The model under review builds one solid part; all positions refer to its coordinate system, in mm. A direction names the side the tool comes from. Round coordinates to 2 decimals unless told otherwise and drop trailing zeros. Write each loop counter-clockwise with the first axis right and the second up, starting at its lowest first coordinate (ties: lowest second). Pieces come first, ordered by that corner, then holes. Notation, with made-up numbers: (46, 79) -> (52, 79) arc R18 cw to (52, 85) -> close; hole circle Ø11 at (39, -32). An arc over 180 degrees is marked (long way). Answer as a JSON object with one key per item and string values. Group by question number.
1) We need section D-D, the plane z = 1.6. Write out the cut boundary in (x, y), then the cut area to 3 significant figures.
2) We need section B-B, the plane z = 0.5. Write out the cut boundary in (x, y).
3) Insertion check: pin 1 Ø3 at (x, z) = (5.5, 0.5) entering from -Y; pin 2 Ø1.1 at (x, z) = (7.54, 0) entering from +Y; pin 3 Ø0.6 at (x, z) = (-9, 0) entering from +Y. Each pin has a flat end and moves straight along its axis. Give the tip position at first contact, or say it passes through.
4) Mouldability with a two-part tool opening along X and no side actions: class faces 4 (the flat face through (11, 5, 0)), 5 (the flat face through (11, 0, 1)), 6 (the flat face through (0, 5, 0)) as pulls with the +X half, pulls with the -X half, needs draft (parallel to the pull), parting line crosses it, or undercut.
5) We need section C-C, the plane y = 2.25. Write out the cut boundary in (x, z) (3 decimals).
6) To check wall thickness, follow probe 1 along X at (y, z) = (1.7, 0) (3 decimals); probe 2 along Z at (x, y) = (-11.5, 3) (3 decimals); probe 3 along Y at (x, z) = (3.5, -1.9). State the ranges of each line that lie inside material, in increasing order. Write a range as [from, to].
7) We need section A-A, the plane y = 6.5. Write out the cut boundary in (x, z) (3 decimals), then the cut area to 3 significant figures.
8) Machinability: for faces 1 (the flat face through (-12, 0, 1)), 2 (the cylindrical face through (-7.628, 6.521, -0.263)), 3 (the cylindrical face through (10.626, 2.465, -0.038)), which of the approach directions +Z, -Z, +X, -X, +Y, -Y give a long, thin tool a straight path to every point of the face, cutting with its end or side? Answer none if there is none.
from build123d import *

# Parameters (mm, degrees)
SKETCH1_R             = 2.875
SKETCH1_R_2           = 0.875
BOSS_EXTRUDE1_DEPTH   = 5
BOSS_EXTRUDE1_2_DEPTH = 5
BOSS_EXTRUDE2_DEPTH   = 3
SKETCH3_R             = 0.875
CUT_EXTRUDE1_DEPTH    = 3


with BuildPart() as part:
    # Sketch1 → Boss-Extrude1 (new body)
    with BuildSketch(Plane(origin=(0, 0, 0), x_dir=(1, 0, 0), z_dir=(0, 1, 0))):
        with Locations((-11.5, 0)):
            Circle(SKETCH1_R)
        with Locations((-11.5, 0)):
            Circle(SKETCH1_R_2, mode=Mode.SUBTRACT)
    extrude(amount=BOSS_EXTRUDE1_DEPTH)



with BuildPart() as body_2:
    # Sketch1 → Boss-Extrude1 2 (new body)
    with BuildSketch(Plane(origin=(0, 0, 0), x_dir=(1, 0, 0), z_dir=(0, 1, 0))):
        with Locations((11.5, 0)):
            Circle(SKETCH1_R)
        with Locations((11.5, 0)):
            Circle(SKETCH1_R_2, mode=Mode.SUBTRACT)
    extrude(amount=BOSS_EXTRUDE1_2_DEPTH)


with BuildPart() as part_1:
    add(part.part)

    add(body_2.part)  # Boss-Extrude2 merges body 2
    # Sketch2 → Boss-Extrude2 (add)
    with BuildSketch(Plane(origin=(0, 5, 0), x_dir=(1, 0, 0), z_dir=(0, 1, 0))):
        with BuildLine():
            ThreePointArc((-10.625, 0), (-10.881281566, 0.618718434), (-11.5, 0.875))
            Line((-11.5, 0.875), (-11.5, -0.875))
            ThreePointArc((-11.5, -0.875), (-10.881281566, -0.618718434), (-10.625, 0))
        make_face()
        with BuildLine():
            Line((-11.5, -0.875), (-11.5, 0.875))
            ThreePointArc((-11.5, 0.875), (-12.375, 0), (-11.5, -0.875))
        make_face()
        with BuildLine():
            ThreePointArc((-8.625, 0), (-9.467068004, 2.032931996), (-11.5, 2.875))
            Line((-11.5, 2.875), (-11.5, 0.875))
            ThreePointArc((-11.5, 0.875), (-10.881281566, 0.618718434), (-10.625, 0))
            ThreePointArc((-10.625, 0), (-10.881281566, -0.618718434), (-11.5, -0.875))
            Line((-11.5, -0.875), (-11.5, -2.875))
            ThreePointArc((-11.5, -2.875), (-9.467068004, -2.032931996), (-8.625, 0))
        make_face()
        with BuildLine():
            Line((-11.5, 0.875), (-11.5, 2.875))
            ThreePointArc((-11.5, 2.875), (-14.375, 0), (-11.5, -2.875))
            Line((-11.5, -2.875), (-11.5, -0.875))
            ThreePointArc((-11.5, -0.875), (-12.375, 0), (-11.5, 0.875))
        make_face()
        with BuildLine():
            Line((11.5, 2.875), (-11.5, 2.875))
            ThreePointArc((-11.5, 2.875), (-9.467068004, 2.032931996), (-8.625, 0))
            ThreePointArc((-8.625, 0), (-9.467068004, -2.032931996), (-11.5, -2.875))
            Line((-11.5, -2.875), (11.5, -2.875))
            ThreePointArc((11.5, -2.875), (8.625, 0), (11.5, 2.875))
        make_face()
        with BuildLine():
            ThreePointArc((14.375, 0), (13.532931996, 2.032931996), (11.5, 2.875))
            Line((11.5, 2.875), (11.5, -2.875))
            ThreePointArc((11.5, -2.875), (13.532931996, -2.032931996), (14.375, 0))
        make_face()
        with BuildLine():
            Line((11.5, -2.875), (11.5, 2.875))
            ThreePointArc((11.5, 2.875), (8.625, 0), (11.5, -2.875))
        make_face()
    extrude(amount=BOSS_EXTRUDE2_DEPTH)

    # Sketch3 → Cut-Extrude1 (cut)
    with BuildSketch(Plane(origin=(0, 8, 0), x_dir=(1, 0, 0), z_dir=(0, 1, 0))):
        with Locations((-8.4626864, 0)):
            Circle(SKETCH3_R)
        with Locations((7.537175494, 0)):
            Circle(SKETCH3_R)
    extrude(amount=-CUT_EXTRUDE1_DEPTH, mode=Mode.SUBTRACT)


solid = part_1.part
Here are the results:
{
 "1": {"outline": "(-13.89, 0) -> (-9.11, 0) -> (-9.11, 5) -> (9.11, 5) -> (9.11, 0) -> (13.89, 0) -> (13.89, 8) -> (-13.89, 8) -> close", "area": "131 mm^2"},
 "2": {"outline": "(-14.33, 0) -> (-12.22, 0) -> (-12.22, 5) -> (-10.78, 5) -> (-10.78, 0) -> (-8.67, 0) -> (-8.67, 5) -> (-9.18, 5) -> (-9.18, 8) -> (-14.33, 8) -> close; (-7.74, 5) -> (6.82, 5) -> (6.82, 8) -> (-7.74, 8) -> close; (8.26, 5) -> (8.67, 5) -> (8.67, 0) -> (10.78, 0) -> (10.78, 5) -> (12.22, 5) -> (12.22, 0) -> (14.33, 0) -> (14.33, 8) -> (8.26, 8) -> close"},
 "3": {"pin 1": "stops at y = 5", "pin 2": "passes through", "pin 3": "stops at y = 5"},
 "4": {"face 4": "undercut", "face 5": "needs draft", "face 6": "undercut"},
 "5": {"outline": "circle Ø5.75 at (-11.5, 0); circle Ø5.75 at (11.5, 0); hole circle Ø1.75 at (-11.5, 0); hole circle Ø1.75 at (11.5, 0)"},
 "6": {"probe 1": "x = [-14.375, -12.375], [-10.625, -8.625], [8.625, 10.625], [12.375, 14.375]", "probe 2": "z = [-2.875, -0.875], [0.875, 2.875]", "probe 3": "y = [5, 8]"},
 "7": {"outline": "(-11.5, -2.875) -> (11.5, -2.875) arc R2.875 ccw to (11.5, 2.875) -> (-11.5, 2.875) arc R2.875 ccw to start; hole circle Ø1.75 at (-8.463, 0); hole circle Ø1.75 at (7.537, 0)", "area": "153 mm^2"},
 "8": {"face 1": "+Z, -Z, +X, -X, -Y", "face 2": "+Y", "face 3": "-Y"}
}
